Design review of the part built by this model. Coordinates are the model's own, in mm. A direction names the side the tool comes from. Give positions to 0.01 mm unless a question says otherwise; leave off trailing zeros. Loops run counter-clockwise (first coordinate to the right, second up) from the corner with the lowest first, then second, coordinate; pieces in that order, holes last. Notation, with made-up numbers: (48, -13) -> (67, -13) arc R26 ccw to (67, 22) -> close; hole circle Ø1 at (-25.75, 32.5). An arc over 180 degrees is marked (long way). Answer in a Markdown table with one row per item. Add a question column.
(1) For pin 1 (2 mm diameter, centred on x = -0.5, z = -0.5, fed in from -Y); pin 2 (1 mm diameter, centred on y = 1, z = -1, fed in from +X); pin 3 (1.6 mm diameter, centred on x = -0.5, z = -4.5, fed in from +Y), all flat-tipped, find the tip position at first contact; note any pin that passes through.
(2) Consider section A-A on z = -4. Write out the cut boundary in (x, y).
(3) For faces 1 (the flat face through (3.29, 0.5, 1.75)), 2 (the cylindrical face through (4.321, 0.246, 2.515)), 3 (the cylindrical face through (-1.341, 0.74, 3.233)), list the 3-axis set-ups (+Z, -Z, +X, -X, +Y, -Y) from which the entire face can be reached by the end or side of a thin tool; tool diameter is ignored.
(4) Draft analysis for pull direction Z (two halves, no side actions). For faces 4 (the flat face through (-1, 2.25, 0)), 5 (the cylindrical face through (-4.34, 0.25, 2.48)), 6 (the flat face through (-3.1, 0.5, 2.2)), state which applies: +Z half, -Z half, draft (parallel to the pull), parting line (faces both ways), or undercut.
(5) Consider section C-C on y = 1.1. Write out the cut boundary in (x, z), then the cut area to 3 significant figures.
(6) For line 1 (X direction, y = 1.05, z = 0); line 2 (Z direction, x = 1.75, y = 1.85), list the stretches that pass through material, from the lowest coordinate up.
from build123d import *
from build123d.topology import SkipClean

# Parameters (mm, degrees)
SKETCH1_R               = 3.5
BOSS_EXTRUDE1_DEPTH     = 2.5
SHELL1_T                = -0.25
SKETCH1_3_R             = 0.375
BOSS_EXTRUDE2_DEPTH     = 0.5
FILLET2_R               = 1
CUT_EXTRUDE1_DEPTH      = 8.133041914
LPATTERN3_COUNT         = 7
LPATTERN3_PITCH         = 0.6
BOSS_EXTRUDE3_START     = -0.25
SKETCH4_R               = 1.25
SKETCH4_R_2             = 0.75
BOSS_EXTRUDE3_DEPTH     = 0.75
FILLET3_R               = 0.2
CUT_EXTRUDE2_DEPTH      = 8.133041914
CUT_EXTRUDE2_DEPTH_BACK = 8.133041914
SKETCH4_2_R             = 0.75


with BuildPart() as part:
    # Sketch1 → Boss-Extrude1 (new body)
    with BuildSketch(Plane(origin=(0, 0, 0), x_dir=(1, 0, 0), z_dir=(0, 1, 0))):
        with Locations(Location((0, 0, 0), (0, 0, 270))):
            Circle(SKETCH1_R)
    extrude(amount=BOSS_EXTRUDE1_DEPTH)

    # Shell1
    shell1_openings = [part.faces().sort_by_distance(p)[0] for p in [
        (0, 0, 0),
    ]]
    offset(amount=SHELL1_T, openings=shell1_openings, kind=Kind.INTERSECTION)

    # Sketch1<3> → Boss-Extrude2 (add)
    # profile 1 of 3: a face of its own
    with BuildSketch(Plane(origin=(0, 0, 0), x_dir=(1, 0, 0), z_dir=(0, 1, 0))):
        with BuildLine():
            Line((3.996834834, -1.444926057), (3.334771827, -1.062683802))
            ThreePointArc((3.334771827, -1.062683802), (3.031088913, -1.75), (2.587697082, -2.356655217))
            Line((2.587697082, -2.356655217), (3.249760089, -2.738897472))
            ThreePointArc((3.249760089, -2.738897472), (4.330127019, -2.5), (3.996834834, -1.444926057))
        make_face()
        with Locations(Location((3.680607966, -2.125, 0), (0, 0, 270))):
            Circle(SKETCH1_3_R, mode=Mode.SUBTRACT)
    # profile 2 of 3: a face of its own
    with BuildSketch(Plane(origin=(0, 0, 0), x_dir=(1, 0, 0), z_dir=(0, 1, 0))):
        with BuildLine():
            ThreePointArc((-0.747074745, 3.419339019), (0, 3.5), (0.747074745, 3.419339019))
            Line((0.747074745, 3.419339019), (0.747074745, 4.183823529))
            ThreePointArc((0.747074745, 4.183823529), (0, 5), (-0.747074745, 4.183823529))
            Line((-0.747074745, 4.183823529), (-0.747074745, 3.419339019))
        make_face()
        with Locations(Location((0, 4.25, 0), (0, 0, 270))):
            Circle(SKETCH1_3_R, mode=Mode.SUBTRACT)
    # profile 3 of 3: a face of its own
    with BuildSketch(Plane(origin=(0, 0, 0), x_dir=(1, 0, 0), z_dir=(0, 1, 0))):
        with BuildLine():
            ThreePointArc((-2.587697082, -2.356655217), (-3.031088913, -1.75), (-3.334771827, -1.062683802))
            Line((-3.334771827, -1.062683802), (-3.996834834, -1.444926057))
            ThreePointArc((-3.996834834, -1.444926057), (-4.330127019, -2.5), (-3.249760089, -2.738897472))
            Line((-3.249760089, -2.738897472), (-2.587697082, -2.356655217))
        make_face()
        with Locations(Location((-3.680607966, -2.125, 0), (0, 0, 270))):
            Circle(SKETCH1_3_R, mode=Mode.SUBTRACT)
    extrude(amount=BOSS_EXTRUDE2_DEPTH)

    # Fillet2
    fillet2_edges = [part.edges().sort_by_distance(p)[0] for p in [
        (0, 2.5, -3.5),
    ]]
    fillet(fillet2_edges, radius=FILLET2_R)

    # Sketch3 → Cut-Extrude1 (cut, symmetric)
    with BuildSketch(Plane(origin=(0, 2.5, 0), x_dir=(1, 0, 0), z_dir=(0, 1, 0))):
        with BuildLine():
            Line((1.625, -2), (1.625, 2))
            ThreePointArc((1.625, 2), (1.8, 2.175), (1.975, 2))
            Line((1.975, 2), (1.975, -2))
            ThreePointArc((1.975, -2), (1.8, -2.175), (1.625, -2))
        make_face()
    cut_extrude1 = extrude(amount=CUT_EXTRUDE1_DEPTH, both=True, mode=Mode.SUBTRACT)

    # LPattern3: Cut-Extrude1 ×7
    with Locations(*[(-i * LPATTERN3_PITCH, 0, 0) for i in range(1, LPATTERN3_COUNT)]):
        add(cut_extrude1, mode=Mode.SUBTRACT)

    # Sketch4 → Boss-Extrude3 (add)
    with BuildSketch(Plane(origin=(0, 2.5, 0), x_dir=(1, 0, 0), z_dir=(0, 1, 0)).offset(BOSS_EXTRUDE3_START)):
        with Locations(Location((0, 0, 0), (0, 0, 81.952153753))):
            Circle(SKETCH4_R)
        with Locations(Location((0, 0, 0), (0, 0, 76.506601178))):
            Circle(SKETCH4_R_2, mode=Mode.SUBTRACT)
    extrude(amount=BOSS_EXTRUDE3_DEPTH)

    # Fillet3
    fillet3_edges = [part.edges().sort_by_distance(p)[0] for p in [
        (-0.175, 3, 1.237689379),
    ]]
    fillet(fillet3_edges, radius=FILLET3_R)

    # Sketch4<2> → Cut-Extrude2 (cut, two sides: drawn at the far end of the back side and taken through both)
    with SkipClean():  # the faces are left unmerged after this step: merging them gives an invalid solid
        with BuildSketch(Plane(origin=(0, 2.5, 0), x_dir=(1, 0, 0), z_dir=(0, 1, 0)).offset(-CUT_EXTRUDE2_DEPTH_BACK)):
            with Locations(Location((0, 0, 0), (0, 0, 270))):
                Circle(SKETCH4_2_R)
        extrude(amount=CUT_EXTRUDE2_DEPTH + CUT_EXTRUDE2_DEPTH_BACK, mode=Mode.SUBTRACT)


solid = part.part
Values follow:
| question | item | result |
|---|---|---|
| 1 | pin 1 | y = 2.25 |
| 1 | pin 2 | x = 3.46 |
| 1 | pin 3 | y = 0.5 |
| 2 | outline | (-0.75, 0) -> (-0.28, 0) -> (-0.28, 0.5) -> (-0.75, 0.5) -> close; (0.28, 0) -> (0.75, 0) -> (0.75, 0.5) -> (0.28, 0.5) -> close |
| 3 | face 1 | +Z, +X, +Y |
| 3 | face 2 | +Y, -Y |
| 3 | face 3 | +Y |
| 4 | face 4 | undercut |
| 4 | face 5 | parting line |
| 4 | face 6 | draft |
| 5 | outline | circle Ø7 at (0, 0); hole circle Ø6.5 at (0, 0) |
| 5 | area | 5.30 mm2 |
| 6 | line 1 | -3.5 to -3.25, 3.25 to 3.5 |
| 6 | line 2 | -2.96 to -2.74, 2.74 to 2.96 |
